Check sheet for the modelled part. Datum: model origin and axes. Units: mm. A direction names the side the tool comes from. Round coordinates to 2 decimals unless told otherwise and drop trailing zeros. Loops run counter-clockwise (first coordinate to the right, second up) from the corner with the lowest first, then second, coordinate; pieces in that order, holes last. Notation, with made-up numbers: (60, -39.5) - (70, -39.5) arc R8 ccw to (70, -26.5) - close; hole circle Ø3 at (0, -3). An arc over 180 degrees is marked (long way). Put each result on its own line as item: value.
```python
from build123d import *

# Parameters (mm, degrees)
SKETCH001_W = 0.5
SKETCH001_H = 0.5
PAD_DEPTH   = 5
FILLET_R    = 2.49


with BuildPart() as part:
    # Sketch → Revolution (revolve)
    with BuildSketch(Plane.XZ):
        with BuildLine():
            Line((0, 0), (2.85, 0))
            Line((2.85, 0), (2.85, 1))
            Line((2.85, 1), (2.5, 1))
            Line((2.5, 1), (2.5, 7.5))
            ThreePointArc((2.5, 7.5), (1.386542, 8.384463), (0, 8.7))
            Line((0, 0), (0, 8.7))
        make_face()
    revolve(axis=Axis((0, 0, 0), (0, 0, 1)))

    # Sketch001 (on Face1 of Revolution) → Pad (new body)
    with BuildSketch(Plane(origin=(0, 0, 0), x_dir=(1, 0, 0), z_dir=(0, 0, -1))):
        with Locations((1.27, 0)):
            Rectangle(SKETCH001_W, SKETCH001_H)
        with Locations((-1.27, 0)):
            Rectangle(SKETCH001_W, SKETCH001_H)
    extrude(amount=PAD_DEPTH)

    # Fillet
    fillet_edges = [part.edges().sort_by_distance(p)[0] for p in [
        (-2.5, 0, 7.5),
    ]]
    fillet(fillet_edges, radius=FILLET_R)


solid = part.part
```
Item 1: Thickness scan on line 1 (Z direction, x = 2.65, y = 0.35); line 2 (Y direction, x = 0.8, z = 4.25); line 3 (X direction, y = -0.4, z = 8). Record the ranges inside material, lowest first. Write a range as from..to.
Filled sheet:
line 1: 0..1
line 2: -2.37..2.37
line 3: -1.69..1.69
Item 2: Go/stop test with flat-tipped pins: pin 1 (2 mm diameter, centred on x = 1, y = 1.5, fed in from -Z); pin 2 (3 mm diameter, centred on x = -1, y = -0.5, fed in from +Z); pin 3 (1.5 mm diameter, centred on x = 0, z = -2, fed in from +Y); pin 4 (2 mm diameter, centred on y = -1, z = -1.5, fed in from -X). Record where each tip stops, or that it passes through.
Filled sheet:
pin 1: z = 0
pin 2: z = 8.7
pin 3: through
pin 4: x = -1.52
Item 3: Tool access check on faces 1 (the cylindrical face through (-2.262, -1.734, 0.507)), 2 (the cylindrical face through (2.385, 0.751, 3.641)). Record the directions out of +Z, -Z, +X, -X, +Y, -Y that give a thin tool (end or side, any length) a straight path to the whole face; none if there is none.
Filled sheet:
face 1: +Z, -Z
face 2: +Z
Item 4: Section check B-B on z = 2. Enter the section's corners in (x, y).
Filled sheet:
outline: circle Ø5 at (0, 0)
Item 5: Section check A-A on z = -2.75. Enter the section's corners in (x, y).
Filled sheet:
outline: (-1.52, -0.25) - (-1.02, -0.25) - (-1.02, 0.25) - (-1.52, 0.25) - close; (1.02, -0.25) - (1.52, -0.25) - (1.52, 0.25) - (1.02, 0.25) - close
